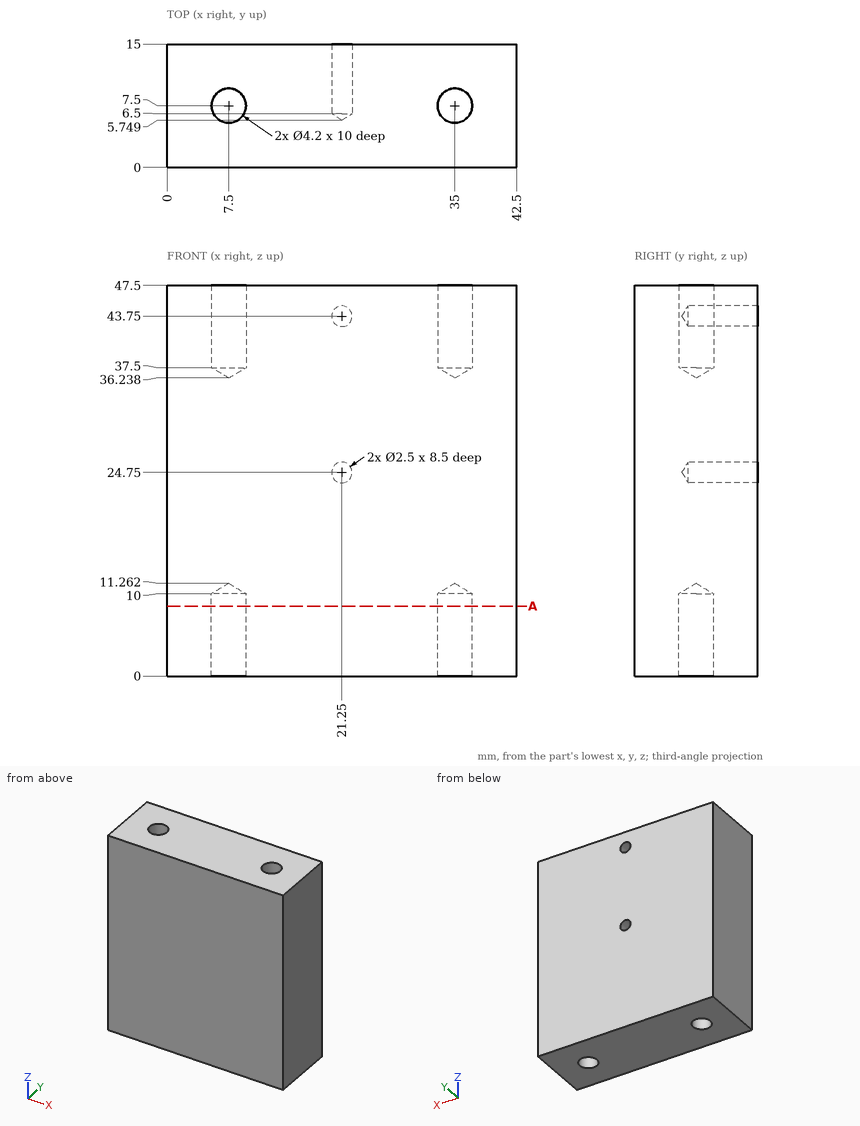
Design review of the part shown in the three views and the two pictorial views. Dimensions are in mm from the part's minimum x, y and z. Give positions to 0.01 mm unless a question says otherwise; leave off trailing zeros. Write each loop counter-clockwise with the first axis right and the second up, starting at its lowest first coordinate (ties: lowest second). Pieces come first, ordered by that corner, then holes.
Item 1: Take a section at A-A (z = 8.5). Give the boundary of the cut face in (x, y), and give its area (3 significant figures).
Item 2: Wall thickness on probe 1 along Z at (x, y) = (21.25, 13); probe 2 along X at (y, z) = (7.5, 2); probe 3 along X at (y, z) = (10, 43.75): over which ranges is each line inside the solid? List them lowest first.
Item 3: Insertion check: P1, Ø4, axis at x = 35, y = 7.5, coming from the -Z side. The pin has a flat end and moves straight along its axis. Give the tip position at first contact, or say it passes through.
Established:
1. outline: (0, 0) - (42.5, 0) - (42.5, 15) - (0, 15) - close; hole circle Ø4.2 at (7.5, 7.5); hole circle Ø4.2 at (35, 7.5)
1. area: 610 mm2
2. probe 1: z = 0 to 23.5, 26 to 42.5, 45 to 47.5
2. probe 2: x = 0 to 5.4, 9.6 to 32.9, 37.1 to 42.5
2. probe 3: x = 0 to 20, 22.5 to 42.5
3. P1: stops at z = 10.06
